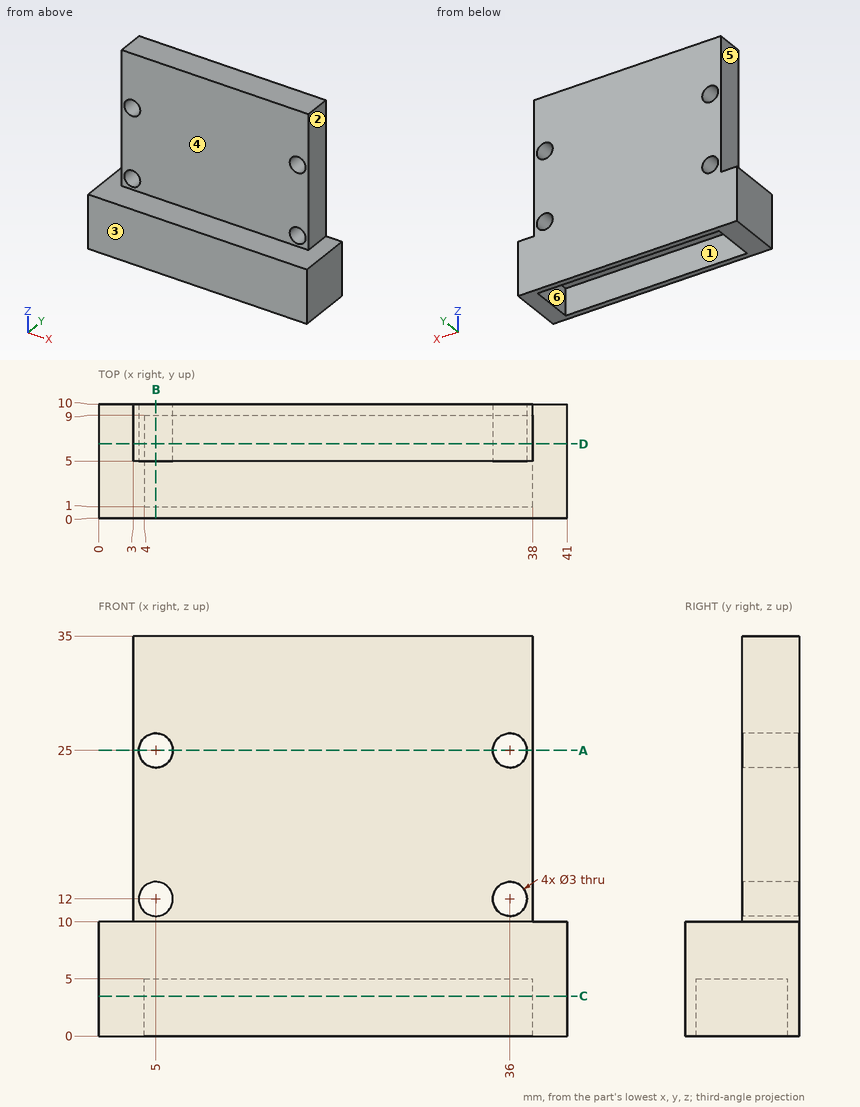
Check sheet for the drawn part. Datum: minimum x, y, z corner. Units: mm. A direction names the side the tool comes from. Coordinates: 2 decimals unless noted, no trailing zeros. Write each loop counter-clockwise with the first axis right and the second up, starting at its lowest first coordinate (ties: lowest second). Pieces come first, ordered by that corner, then holes. Notation, with made-up numbers: M 16.25,47.25 L 75.25,47.25 A25 cw 75.25,72.25 Z; hole C -7.5,-32 d2. An arc over 180 degrees is marked long. One line per item, written item: value.
Item 1: Section check B-B, the plane x = 5. Record the boundary of the cut face in (y, z).
Check sheet entries:
outline: M 0,0 L 1,0 L 1,5 L 9,5 L 9,0 L 10,0 L 10,10.5 L 5,10.5 L 5,10 L 0,10 Z; M 5,13.5 L 10,13.5 L 10,23.5 L 5,23.5 Z; M 5,26.5 L 10,26.5 L 10,35 L 5,35 Z
Item 2: Gauge pin test, flat ends, axial feed: pin 1 Ø2.5 at (x, y) = (25.5, 4) entering from -Z; pin 2 Ø7.5 at (x, z) = (22.5, 26.5) entering from -Y; pin 3 Ø2.5 at (y, z) = (7.5, 20.5) entering from +X. Record the tip position at first contact, or that the pin passes through.
Check sheet entries:
pin 1: stops at z = 5
pin 2: stops at y = 5
pin 3: stops at x = 38
Item 3: Section check C-C, the plane z = 3.5. Record the boundary of the cut face in (x, y), plus the area to 3 significant figures.
Check sheet entries:
outline: M 0,0 L 41,0 L 41,10 L 0,10 Z; hole M 4,1 L 38,1 L 38,9 L 4,9 Z
area: 138 mm^2
Item 4: Scan lines: line 1 along Z through (x, y) = (36, 7.7); line 2 along X through (y, z) = (8.2, 25); line 3 along Y through (x, z) = (14.5, 3). Record each from-to range of solid material in increasing order.
Check sheet entries:
line 1: z = 5 to 10.5, 13.5 to 23.5, 26.5 to 35
line 2: x = 3 to 3.5, 6.5 to 34.5, 37.5 to 38
line 3: y = 0 to 1, 9 to 10
Item 5: Section check D-D, the plane y = 6.5. Record the boundary of the cut face in (x, z).
Check sheet entries:
outline: M 0,0 L 4,0 L 4,5 L 38,5 L 38,0 L 41,0 L 41,10 L 38,10 L 38,35 L 3,35 L 3,10 L 0,10 Z; hole C 5,12 d3; hole C 5,25 d3; hole C 36,12 d3; hole C 36,25 d3
Item 6: Section check A-A, the plane z = 25. Record the boundary of the cut face in (x, y).
Check sheet entries:
outline: M 3,5 L 3.5,5 L 3.5,10 L 3,10 Z; M 6.5,5 L 34.5,5 L 34.5,10 L 6.5,10 Z; M 37.5,5 L 38,5 L 38,10 L 37.5,10 Z
Item 7: Mould release check, pull along Y, two halves, no side actions. Record for the marked faces 1, 2 and 3: pulls with the +Y half, pulls with the -Y half, needs draft (parallel to the pull), parting line crosses it, or undercut.
Check sheet entries:
face 1: undercut
face 2: needs draft
face 3: pulls with the -Y half
Item 8: Access from +Z, -Z, +X, -X, +Y, -Y to the whole of each face (thin tool, end or side, straight path). Record for the marked faces 4, 5 and 6.
Check sheet entries:
face 4: +Z, +X, -X, -Y
face 5: +Z, -X, +Y, -Y
face 6: -Z
